Part model, mm, in its own coordinate system. Coordinates: 2 decimals unless noted, no trailing zeros. Loops run counter-clockwise (first coordinate to the right, second up) from the corner with the lowest first, then second, coordinate; pieces in that order, holes last. Notation, with made-up numbers: (31.25, 19) - (74.25, 19) arc R5 cw to (74.25, 23) - close; hole circle Ø11 at (-7, -30.75). An arc over 180 degrees is marked (long way). Use a Markdown table: item, result. Add a question column.
1. Band-saw the part on C-C, the plane x = -53.5. Give the cut face in (y, z) (3 decimals).
2. Band-saw the part on A-A, the plane y = 1. Give the cut face in (x, z) (1 decimal), plus the area to 3 significant figures.
3. Wall check: probe 1 along X at (y, z) = (1, 2.2) (1 decimal); probe 2 along Y at (x, z) = (-36.5, 1.05) (3 decimals); probe 3 along X at (y, z) = (-21.5, 2.65). Give the ranges that are in metal, low to high. Write a range as [from, to].
4. Band-saw the part on B-B, the plane x = 41. Give the cut face in (y, z) (3 decimals).
5. Band-saw the part on D-D, the plane z = 1.25. Count the separate pieces of the cut face and the enclosed holes in it, plus the area to 3 significant figures.
6. Drop flat-ended pins along their axis: pin 1 (2 mm diameter, centred on y = 36, z = 2, fed in from -X); pin 2 (3.5 mm diameter, centred on x = -53.71, y = 29.59, fed in from +Z); pin 3 (2 mm diameter, centred on y = 35.5, z = 1.5, fed in from +X). Give the stop position or say it passes through.
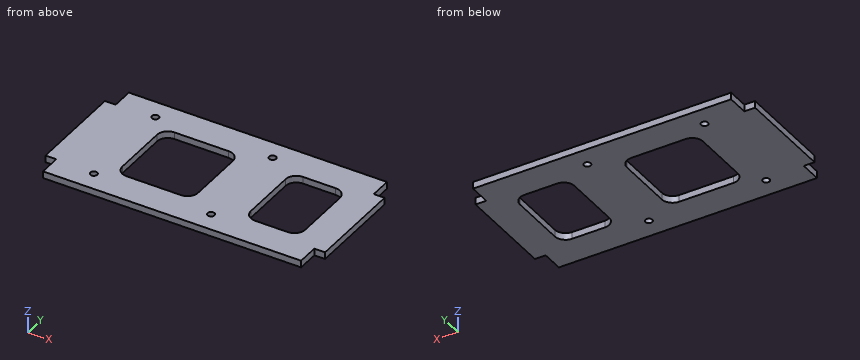
from build123d import *

# Parameters (mm, degrees)
SKETCH1_R           = 2.032
BOSS_EXTRUDE1_DEPTH = 4.064


with BuildPart() as part:
    # Sketch1 → Boss-Extrude1 (new body)
    with BuildSketch(Plane.XY):
        Polygon((75.8825, -41.275), (-76.5175, -41.275), (-76.5175, -28.575), (-82.8675, -28.575), (-82.8675, 28.575), (-76.5175, 28.575), (-76.5175, 41.275), (75.8825, 41.275), (75.8825, 28.575), (82.2325, 28.575), (82.2325, -28.575), (75.8825, -28.575), align=None)
        with Locations((-53.709797321, 29.591)):
            Circle(SKETCH1_R, mode=Mode.SUBTRACT)
        with Locations((15.5575, 29.591)):
            Circle(SKETCH1_R, mode=Mode.SUBTRACT)
        with Locations((-53.709797321, -29.591)):
            Circle(SKETCH1_R, mode=Mode.SUBTRACT)
        with Locations((15.5575, -29.591)):
            Circle(SKETCH1_R, mode=Mode.SUBTRACT)
        with BuildLine():
            Line((56.8325, 22.987), (37.465, 22.987))
            ThreePointArc((37.465, 22.987), (32.974871939, 21.127128061), (31.115, 16.637))
            Line((31.115, 16.637), (31.115, -16.637))
            ThreePointArc((31.115, -16.637), (32.974871939, -21.127128061), (37.465, -22.987))
            Line((37.465, -22.987), (56.8325, -22.987))
            ThreePointArc((56.8325, -22.987), (61.322628061, -21.127128061), (63.1825, -16.637))
            Line((63.1825, -16.637), (63.1825, 16.637))
            ThreePointArc((63.1825, 16.637), (61.322628061, 21.127128061), (56.8325, 22.987))
        make_face(mode=Mode.SUBTRACT)
        with BuildLine():
            Line((-6.35, 22.987), (-38.4175, 22.987))
            ThreePointArc((-38.4175, 22.987), (-42.907628061, 21.127128061), (-44.7675, 16.637))
            Line((-44.7675, 16.637), (-44.7675, -16.637))
            ThreePointArc((-44.7675, -16.637), (-42.907628061, -21.127128061), (-38.4175, -22.987))
            Line((-38.4175, -22.987), (-6.35, -22.987))
            ThreePointArc((-6.35, -22.987), (-1.859871939, -21.127128061), (0, -16.637))
            Line((0, -16.637), (0, 16.637))
            ThreePointArc((0, 16.637), (-1.859871939, 21.127128061), (-6.35, 22.987))
        make_face(mode=Mode.SUBTRACT)
    extrude(amount=BOSS_EXTRUDE1_DEPTH)


solid = part.part
Geometry check:
| question | item | result |
|---|---|---|
| 1 | outline | (-41.275, 0) - (-31.612, 0) - (-31.612, 4.064) - (-41.275, 4.064) - close; (-27.57, 0) - (27.57, 0) - (27.57, 4.064) - (-27.57, 4.064) - close; (31.612, 0) - (41.275, 0) - (41.275, 4.064) - (31.612, 4.064) - close |
| 2 | outline | (-82.9, 0) - (-44.8, 0) - (-44.8, 4.1) - (-82.9, 4.1) - close; (0, 0) - (31.1, 0) - (31.1, 4.1) - (0, 4.1) - close; (63.2, 0) - (82.2, 0) - (82.2, 4.1) - (63.2, 4.1) - close |
| 2 | area | 359 mm^2 |
| 3 | probe 1 | x = [-82.9, -44.8], [0, 31.1], [63.2, 82.2] |
| 3 | probe 2 | y = [-41.275, -22.987], [22.987, 41.275] |
| 3 | probe 3 | x = [-82.87, -42.5], [-2.27, 33.38], [60.92, 82.23] |
| 4 | outline | (-41.275, 0) - (-22.987, 0) - (-22.987, 4.064) - (-41.275, 4.064) - close; (22.987, 0) - (41.275, 0) - (41.275, 4.064) - (22.987, 4.064) - close |
| 5 | separate pieces | 1 |
| 5 | enclosed holes | 6 |
| 5 | area | 9,790 mm^2 |
| 6 | pin 1 | stops at x = -76.52 |
| 6 | pin 2 | passes through |
| 6 | pin 3 | stops at x = 75.88 |
